```python
from build123d import *

# Parameters (mm, degrees)
SKETCH1_R      = 1.3716
SKETCH1_R_2    = 1.905
EXTRUDE1_DEPTH = 12.7
SKETCH2_R      = 2.032
EXTRUDE2_DEPTH = 9.652


with BuildPart() as part:
    # Sketch1 → Extrude1 (new body)
    with BuildSketch(Plane.XY):
        with BuildLine():
            Line((-44.40070708, 58.959918893), (-23.474438879, 34.429033799))
            ThreePointArc((-23.474438879, 34.429033799), (-22.79815009, 33.273999736), (-22.563049012, 31.956351187))
            Line((-22.563049012, 31.956351187), (-22.563049012, 17.553595327))
            ThreePointArc((-22.563049012, 17.553595327), (-23.678972175, 14.85951849), (-26.373049012, 13.743595327))
            Line((-26.373049012, 13.743595327), (-31.554570289, 13.743595327))
            ThreePointArc((-31.554570289, 13.743595327), (-36.166042792, 9.132122824), (-31.554570289, 4.520650321))
            Line((-31.554570289, 4.520650321), (-26.373049012, 4.520650321))
            ThreePointArc((-26.373049012, 4.520650321), (-23.678972175, 3.404727157), (-22.563049012, 0.710650321))
            Line((-22.563049012, 0.710650321), (-22.563049012, -1.885593273))
            ThreePointArc((-22.563049012, -1.885593273), (-23.678972175, -4.579670109), (-26.373049012, -5.695593273))
            Line((-26.373049012, -5.695593273), (-34.251425283, -5.695593273))
            Line((-34.251425283, -5.695593273), (-34.251425283, -12.452071481))
            Line((-34.251425283, -12.452071481), (34.251425283, -12.452071481))
            Line((34.251425283, -12.452071481), (34.251425283, -5.695593273))
            Line((34.251425283, -5.695593273), (26.373049012, -5.695593273))
            ThreePointArc((26.373049012, -5.695593273), (23.678972175, -4.579670109), (22.563049012, -1.885593273))
            Line((22.563049012, -1.885593273), (22.563049012, 0.710650321))
            ThreePointArc((22.563049012, 0.710650321), (23.678972175, 3.404727157), (26.373049012, 4.520650321))
            Line((26.373049012, 4.520650321), (31.554570289, 4.520650321))
            ThreePointArc((31.554570289, 4.520650321), (36.166042792, 9.132122824), (31.554570289, 13.743595327))
            Line((31.554570289, 13.743595327), (26.373049012, 13.743595327))
            ThreePointArc((26.373049012, 13.743595327), (23.678972175, 14.85951849), (22.563049012, 17.553595327))
            Line((22.563049012, 17.553595327), (22.563049012, 31.956351187))
            ThreePointArc((22.563049012, 31.956351187), (22.79815009, 33.273999736), (23.474438879, 34.429033799))
            Line((23.474438879, 34.429033799), (44.40070708, 58.959918893))
            ThreePointArc((44.40070708, 58.959918893), (43.861334165, 65.761850412), (37.059402646, 65.222477498))
            Line((37.059402646, 65.222477498), (18.05525325, 42.944802345))
            ThreePointArc((18.05525325, 42.944802345), (16.752760164, 41.957931463), (15.156643118, 41.607484957))
            Line((15.156643118, 41.607484957), (-15.156643118, 41.607484957))
            ThreePointArc((-15.156643118, 41.607484957), (-16.752760164, 41.957931463), (-18.05525325, 42.944802345))
            Line((-18.05525325, 42.944802345), (-37.059402646, 65.222477498))
            ThreePointArc((-37.059402646, 65.222477498), (-43.861334165, 65.761850412), (-44.40070708, 58.959918893))
        make_face()
        with Locations((-40.730054863, 62.091198195)):
            Circle(SKETCH1_R, mode=Mode.SUBTRACT)
        with Locations(Location((31.554570289, 9.132122824, 0), (0, 0, 180))):
            Circle(SKETCH1_R_2, mode=Mode.SUBTRACT)
        with Locations(Location((40.730054863, 62.091198195, 0), (0, 0, 180))):
            Circle(SKETCH1_R, mode=Mode.SUBTRACT)
        with Locations((-31.554570289, 8.979309022)):
            Circle(SKETCH1_R_2, mode=Mode.SUBTRACT)
        with BuildLine():
            Line((-13.673049012, 32.09814334), (13.673049012, 32.09814334))
            ThreePointArc((13.673049012, 32.09814334), (16.367125848, 30.982220177), (17.483049012, 28.28814334))
            Line((17.483049012, 28.28814334), (17.483049012, -4.832071481))
            ThreePointArc((17.483049012, -4.832071481), (16.367125848, -7.526148317), (13.673049012, -8.642071481))
            Line((13.673049012, -8.642071481), (-13.673049012, -8.642071481))
            ThreePointArc((-13.673049012, -8.642071481), (-16.367125848, -7.526148317), (-17.483049012, -4.832071481))
            Line((-17.483049012, -4.832071481), (-17.483049012, 28.28814334))
            ThreePointArc((-17.483049012, 28.28814334), (-16.367125848, 30.982220177), (-13.673049012, 32.09814334))
        make_face(mode=Mode.SUBTRACT)
    extrude(amount=EXTRUDE1_DEPTH)

    # Sketch2 → Extrude2 (cut)
    with BuildSketch(Plane.XZ.offset(12.452071481)):
        with Locations(Location((28.407237147, 6.35, 0), (0, 0, 270))):
            Circle(SKETCH2_R)
        with Locations(Location((-28.407237147, 6.35, 0), (0, 0, 270))):
            Circle(SKETCH2_R)
    extrude(amount=-EXTRUDE2_DEPTH, mode=Mode.SUBTRACT)


solid = part.part
```
Can you work these out from the model? Positions are in its coordinate system, mm. A direction names the side the tool comes from. Give positions to 0.01 mm unless a question says otherwise; leave off trailing zeros. Loops run counter-clockwise (first coordinate to the right, second up) from the corner with the lowest first, then second, coordinate; pieces in that order, holes last. Notation, with made-up numbers: M 3.25,-31 L 17.25,-31 A33 ccw 17.25,3 Z; hole C 82.5,55.25 d7. An arc over 180 degrees is marked long. Use one line per item in the form item = value. Start each with the question number.
(1) I'm going to push flat-ended pins straight in: P1, Ø4, axis at x = -4.5, z = 4.5, coming from the +Y side; P2, Ø0.8, axis at y = -0.5, z = 8.5, coming from the +X side; P3, Ø3, axis at x = 40.73, y = 62.09, coming from the +Z side; P4, Ø4, axis at y = 38, z = 4.5, coming from the +X side. Where does each tip first touch, or does it pass through?
(2) I want a section at A-A, the plane x = 1. Write out the boundary of the cut face in (y, z).
(3) Thinking about a two-plate mould opening in X: for faces 5 (the cylindrical face through (43.941, 65.692, 6.261)), 6 (the flat face through (29, 4.521, 6)), 7 (the flat face through (33.79, 46.52, 6.26)), 8 (the cylindrical face through (-33.066, 7.82, 6.261)), which applies, released by +X, released by -X, zero draft, split by the parting line, or undercut?
(4) On a 3-axis mill with a long thin cutter (end or side, diameter ignored), from which of +Z, -Z, +X, -X, +Y, -Y can I reach the whole of each face in a straight line? I mean faces 1 (the cylindrical face through (23.7, -4.6, 6.3)), 2 (the flat face through (0, 32.098, 6)), 3 (the flat face through (-27.4, 53.9, 6.3)), 4 (the flat face through (-22.563, 25, 6)). Say none if no direction works.
(5) Please list where these lines run through material, in increasing order: line 1 (Y direction, x = 6, z = 5.5); line 2 (X direction, y = -8.25, z = 6.35); line 3 (Y direction, x = -30, z = 6).
(6) I want a section at D-D, the plane z = 6.35. State how many separate pieces and enclosed holes the cut face has, and give its area (3 significant figures).
(7) I want a section at C-C, the plane x = -25. Write out the boundary of the cut face in (y, z).
(8) I want a section at B-B, the plane y = 50.5. Write out the boundary of the cut face in (x, z).
Worked out:
q1.P1 = 41.61
q1.P2 = 22.56
q1.P3 = 12.7
q1.P4 = 28.23
q2.outline = M -12.45,0 L -8.64,0 L -8.64,12.7 L -12.45,12.7 Z; M 32.1,0 L 41.61,0 L 41.61,12.7 L 32.1,12.7 Z
q3.face_5 = undercut
q3.face_6 = zero draft
q3.face_7 = released by +X
q3.face_8 = undercut
q4.face_1 = +Z, -Z, +X
q4.face_2 = +Z, -Z
q4.face_3 = +Z, -Z, +Y
q4.face_4 = +Z, -Z, -X
q5.line_1 = -12.45 to -8.64, 32.1 to 41.61
q5.line_2 = -34.25 to -30.44, -26.38 to -15.36, 15.36 to 26.38, 30.44 to 34.25
q5.line_3 = 4.52 to 7.88, 10.08 to 13.74, 42.08 to 56.95
q6.separate_pieces = 3
q6.enclosed_holes = 5
q6.area = 2,000 mm²
q7.outline = M -12.45,0 L -5.44,0 L -5.44,12.7 L -12.45,12.7 Z; M 4.26,0 L 14,0 L 14,12.7 L 4.26,12.7 Z; M 36.22,0 L 51.09,0 L 51.09,12.7 L 36.22,12.7 Z
q8.outline = M -37.18,0 L -24.5,0 L -24.5,12.7 L -37.18,12.7 Z; M 24.5,0 L 37.18,0 L 37.18,12.7 L 24.5,12.7 Z
